Autodesk Inventor part; units mm, degrees
ref_plane "YZ Plane" through (0, 0, 0) normal (1, 0, 0) x (0, 1, 0)
ref_plane "XZ Plane" through (0, 0, 0) normal (0, 1, 0) x (-1, 0, 0)
ref_plane "XY Plane" through (0, 0, 0) normal (0, 0, 1) x (1, 0, 0)
sketch "Sketch1" plane through (0, 0, 0) normal (1, 0, 0) x (0, 1, 0)
  line L0 (12.5, 0) -> (-12.5, 0)
  line L1 (12.5, 0) -> (7.5, 0)
  line L2 (7.5, 0) -> (7.5, 20)
  line L3 (7.5, 20) -> (8.5, 20)
  line L4 (12.5, 16) -> (12.5, 0)
  line L5 (12.5, 20) -> (0, 20)
  line L6 (0, 20) -> (0, 15)
  line L7 (0, 15) -> (12.5, 15)
  line L8 (12.5, 15) -> (12.5, 20)
  arc A0 (12.5, 16) -> (8.5, 20) centre (8.5, 16) ccw
  line L9 (0, 15) -> (2.9, 15)
  line L10 (2.9, 15) -> (2.9, 1)
  line L11 (2.9, 1) -> (7.5, 1)
  line L12 (12.5, 0) -> (12.5, 0.5)
  line L13 (12.5, 0.5) -> (7.5, 0.5)
  line L14 (0, 15) -> (0.5, 15)
  line L15 (0.5, 15) -> (0.5, 7)
  line L16 (0.5, 7) -> (0, 7)
  line L17 (0, 7) -> (0, 15)
  point P0 (0, 0)
  dimension "d0" = 5
  dimension "d1" = 20
  dimension "d2" = 5
  dimension "d3" = 4
  dimension "d5" = 14
  dimension "d6" = 0.5
  dimension "d7" = 0.5
  dimension "d8" = 8
revolve "Revolution1" add sketch "Sketch1" angle 360 about axis through (0, 0, 7) along (0, 0, 1) contours L13 L2 L7 L4 | L7 L2 L3 A0 L4 | L11 L10 L7 L2 | L7 L6 L5 L2
sketch "Sketch2" plane through (0, 0, 15) normal (0, 0, -1) x (-1, 0, 0)
  line L0 (0.5, 5) -> (-0.5, 5)
  line L1 (-0.5, 5) -> (-0.5, -5)
  line L2 (-0.5, -5) -> (0.5, -5)
  line L3 (0.5, -5) -> (0.5, 5)
  line L4 (0.5, 5) -> (-0.5, -5) construction
  line L5 (-0.5, 5) -> (0.5, -5) construction
  point P0 (0, 0)
  dimension "d10" = 1
  dimension "d11" = 10
extrude "Extrusion1" add sketch "Sketch2" along normal blind 8
properties part number "Brightness"
For this review, take the finished solid that the model builds, in its own axes (mm). A direction names the side the tool comes from. Round coordinates to 2 decimals unless told otherwise and drop trailing zeros. Write each loop counter-clockwise with the first axis right and the second up, starting at its lowest first coordinate (ties: lowest second). Pieces come first, ordered by that corner, then holes. Notation, with made-up numbers: (25.5, 20.5) -> (61.5, 20.5) arc R23 cw to (61.5, 51.5) -> close; hole circle Ø6 at (-16.5, -9). An arc over 180 degrees is marked (long way). Use one line per item in the form item = value.
Q1. Consider section D-D (z = 5.75). State the section outline as (x, y) points.
Resolved:
outline = circle Ø25 at (0, 0); hole circle Ø5.8 at (0, 0)
Q2. To check wall thickness, follow probe 1 along Y at (x, z) = (0, 5.25); probe 2 along X at (y, z) = (0, 0.8); probe 3 along X at (y, z) = (2.25, 12). State the ranges of each line that lie inside material, in increasing order. Write a range as from..to.
Resolved:
probe_1 = -12.5..-2.9, 2.9..12.5
probe_2 = -12.5..-7.5, 7.5..12.5
probe_3 = -12.3..-1.83, -0.5..0.5, 1.83..12.3
Q3. Machinability: for faces 4 (the flat face through (0, 0, 20)), 5 (the flat face through (-1, 0, 15)), which of the approach directions +Z, -Z, +X, -X, +Y, -Y give a long, thin tool a straight path to every point of the face, cutting with its end or side? Answer none if there is none.
Resolved:
face_4 = +Z, +X, -X, +Y, -Y
face_5 = -Z
Q4. The part is to be moulded in two halves that separate along Y. For faces 1 (the flat face through (8, 0, 0.5)), 2 (the cylindrical face through (3.755, 11.923, 8.142)), 3 (the flat face through (3.2, -0.1, 1)), say which applies: released by +Y, released by -Y, zero draft, split by the parting line, or undercut.
Resolved:
face_1 = zero draft
face_2 = split by the parting line
face_3 = undercut
Q5. Clearance check with flat-ended pins moving along their axes: pin 1 Ø1.2 at (x, y) = (2.5, 0) entering from -Z; pin 2 Ø2 at (y, z) = (4, 5) entering from +X; pin 3 Ø0.7 at (x, y) = (-1.5, -0.5) entering from -Z. State where each tip first meets the part, or that it passes through.
Resolved:
pin_1 = 1
pin_2 = 12.13
pin_3 = 15
Q6. Consider section B-B (x = 0). State the section outline as (y, z) points.
Resolved:
outline = (-12.5, 0.5) -> (-7.5, 0.5) -> (-7.5, 1) -> (-2.9, 1) -> (-2.9, 7) -> (2.9, 7) -> (2.9, 1) -> (7.5, 1) -> (7.5, 0.5) -> (12.5, 0.5) -> (12.5, 16) arc R4 ccw to (8.5, 20) -> (-8.5, 20) arc R4 ccw to (-12.5, 16) -> close
Q7. Consider section A-A (z = 13.5). State the section outline as (x, y) points, then the cut area to 3 significant figures.
Resolved:
outline = circle Ø25 at (0, 0); hole (-0.5, -2.86) -> (-0.5, 2.86) arc R2.9 ccw to start; hole (0.5, -2.86) arc R2.9 ccw to (0.5, 2.86) -> close
area = 470 mm²
Q8. Consider section C-C (y = 0). State the section outline as (x, z) points.
Resolved:
outline = (-12.5, 0.5) -> (-7.5, 0.5) -> (-7.5, 1) -> (-2.9, 1) -> (-2.9, 15) -> (-0.5, 15) -> (-0.5, 7) -> (0.5, 7) -> (0.5, 15) -> (2.9, 15) -> (2.9, 1) -> (7.5, 1) -> (7.5, 0.5) -> (12.5, 0.5) -> (12.5, 16) arc R4 ccw to (8.5, 20) -> (-8.5, 20) arc R4 ccw to (-12.5, 16) -> close
